Work out the finished part from the listing and answer in its coordinate system (mm). Coordinates: 2 decimals unless noted, no trailing zeros. Use a Markdown table: item, result.
from build123d import *

# Parameters (mm, degrees)
F0_W     = 32.9184010625
F0_H     = 33.8327996433
F1_DEPTH = 25.4
F2_R     = 9.6783003352
F3_DEPTH = 0.508
F3_TAPER = -30


with BuildPart() as f1:
    # F0 (on Front) → F1 (new body, symmetric)
    with BuildSketch(Plane.XZ):
        Rectangle(F0_W, F0_H)
    extrude(amount=F1_DEPTH, both=True)

    # F2 (on face) → F3 (cut)
    with BuildSketch(Plane.XY.offset(16.9163998216)):
        Circle(F2_R)
    extrude(amount=-F3_DEPTH, taper=F3_TAPER, mode=Mode.SUBTRACT)


solid = f1.part
(1) A straight line is drawn through the part: L1, parallel to Z at x = 3, y = -9. Find the intervals that lie inside material, in ascending order.
Conclusion:
| item | result |
|---|---|
| L1 | -16.92 to 16.41 |
(2) Determine the mould class of faces 1 (the flat face through (0, -25.4, 0)), 2 (the flat face through (0, 25.4, 0)), 3 (the flat face through (0, 0, 16.408)), 4 (the flat face through (16.459, 0, 0)) for opening direction Y: pulls with the +Y half, pulls with the -Y half, needs draft (parallel to the pull), parting line crosses it, or undercut.
Conclusion:
| item | result |
|---|---|
| face 1 | pulls with the -Y half |
| face 2 | pulls with the +Y half |
| face 3 | undercut |
| face 4 | needs draft |
(3) Given P1, Ø3, axis at x = -6.5, y = 3, coming from the +Z side, flat-ended and moving along its own axis, determine where the tip first touches the part or whether it passes through.
Conclusion:
| item | result |
|---|---|
| P1 | z = 16.41 |
